Check sheet for the modelled part. Datum: model origin and axes. Units: mm. Face numbers are marked on the shaded views. A direction names the side the tool comes from. Coordinates: 2 decimals unless noted, no trailing zeros. Write each loop counter-clockwise with the first axis right and the second up, starting at its lowest first coordinate (ties: lowest second). Pieces come first, ordered by that corner, then holes. Notation, with made-up numbers: (52, 51) - (90, 51) arc R30 ccw to (90, 86) - close; hole circle Ø2 at (30, 54). An arc over 180 degrees is marked (long way). Answer as CSV lines item,"result". Start each with the question number.
from build123d import *

# Parameters (mm, degrees)
SKETCH2_W           = 38.1
SKETCH2_H           = 38.1
BOSS_EXTRUDE1_DEPTH = 5.08
SKETCH3_W           = 22.0218
SKETCH3_H           = 38.1
BOSS_EXTRUDE2_DEPTH = 5.08
SKETCH4_W           = 22.0218
SKETCH4_H           = 38.1
BOSS_EXTRUDE3_DEPTH = 5.08
SKETCH5_W           = 38.1
SKETCH5_H           = 38.1
BOSS_EXTRUDE4_DEPTH = 5.08
SKETCH6_R           = 4.826
CUT_EXTRUDE1_DEPTH  = 87.664926553
SKETCH7_R           = 4.826
CUT_EXTRUDE2_DEPTH  = 87.664926553
FILLET1_R           = 2.54
FILLET2_R           = 2.54
FILLET3_R           = 2.54
FILLET4_R           = 2.54
FILLET5_R           = 2.54


with BuildPart() as part:
    # Sketch2 → Boss-Extrude1 (new body)
    with BuildSketch(Plane.XY):
        with Locations((19.05, 19.05)):
            Rectangle(SKETCH2_W, SKETCH2_H)
    extrude(amount=-BOSS_EXTRUDE1_DEPTH)

    # Sketch3 → Boss-Extrude2 (add)
    with BuildSketch(Plane(origin=(38.1, 0, 0), x_dir=(0, 0, -1), z_dir=(1, 0, 0))):
        with Locations((11.0109, 19.05)):
            Rectangle(SKETCH3_W, SKETCH3_H)
    extrude(amount=-BOSS_EXTRUDE2_DEPTH)

    # Sketch4 → Boss-Extrude3 (add)
    with BuildSketch(Plane(origin=(0, 0, -22.0218), x_dir=(-1, 0, 0), z_dir=(0, 0, -1))):
        with Locations((-44.0309, 19.05)):
            Rectangle(SKETCH4_W, SKETCH4_H)
    extrude(amount=-BOSS_EXTRUDE3_DEPTH)

    # Sketch5 → Boss-Extrude4 (add)
    with BuildSketch(Plane(origin=(55.0418, 0, 0), x_dir=(0, 0, -1), z_dir=(1, 0, 0))):
        with Locations((35.9918, 19.05)):
            Rectangle(SKETCH5_W, SKETCH5_H)
    extrude(amount=-BOSS_EXTRUDE4_DEPTH)

    # Sketch6 → Cut-Extrude1 (cut, through all)
    with BuildSketch(Plane(origin=(55.0418, 0, 0), x_dir=(0, 0, -1), z_dir=(1, 0, 0))):
        with Locations((39.8018, 28.575)):
            Circle(SKETCH6_R)
        with Locations(Location((39.8018, 9.525, 0), (0, 0, 180))):
            Circle(SKETCH6_R)
    extrude(amount=-CUT_EXTRUDE1_DEPTH, mode=Mode.SUBTRACT)

    # Sketch7 → Cut-Extrude2 (cut, through all)
    with BuildSketch(Plane.XY):
        with Locations((15.24, 28.575)):
            Circle(SKETCH7_R)
        with Locations(Location((15.24, 9.525, 0), (0, 0, 180))):
            Circle(SKETCH7_R)
    extrude(amount=-CUT_EXTRUDE2_DEPTH, mode=Mode.SUBTRACT)

    # Fillet1
    fillet1_edges = [part.edges().sort_by_distance(p)[0] for p in [
        (49.9618, 19.05, -55.0418),
    ]]
    fillet(fillet1_edges, radius=FILLET1_R)

    # Fillet2
    fillet2_edges = [part.edges().sort_by_distance(p)[0] for p in [
        (49.9618, 19.05, -22.0218),
    ]]
    fillet(fillet2_edges, radius=FILLET2_R)

    # Fillet3
    fillet3_edges = [part.edges().sort_by_distance(p)[0] for p in [
        (33.02, 19.05, -22.0218),
    ]]
    fillet(fillet3_edges, radius=FILLET3_R)

    # Fillet4
    fillet4_edges = [part.edges().sort_by_distance(p)[0] for p in [
        (33.02, 19.05, -5.08),
    ]]
    fillet(fillet4_edges, radius=FILLET4_R)

    # Fillet5
    fillet5_edges = [part.edges().sort_by_distance(p)[0] for p in [
        (0, 19.05, -5.08),
    ]]
    fillet(fillet5_edges, radius=FILLET5_R)


solid = part.part
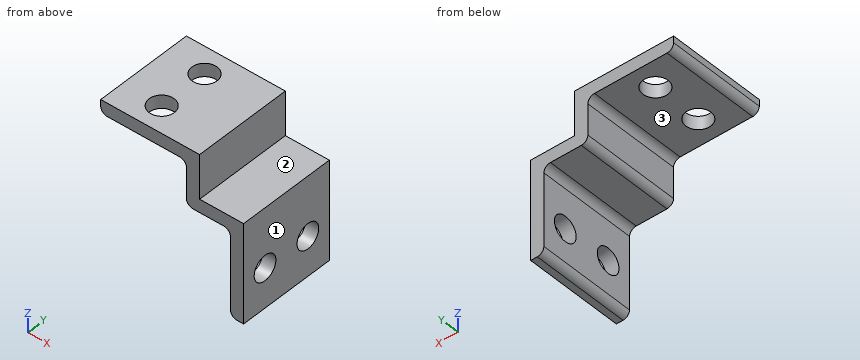
(1) Tool access check on the marked faces 1, 2 and 3. Record the directions out of +Z, -Z, +X, -X, +Y, -Y that give a thin tool (end or side, any length) a straight path to the whole face; none if there is none.
(2) Cross-section at B-B on y = 36. Record the boundary of the cut face in (x, z), plus the area to 3 significant figures.
(3) Cross-section at A-A on x = 15.24. Record the boundary of the cut face in (y, z), plus the area to 3 significant figures.
(4) Go/stop test with flat-tipped pins: P1, Ø12, axis at x = 44, z = -11, coming from the +Y side; P2, Ø12, axis at x = 32, y = 21.5, coming from the -Z side; P3, Ø7.5, axis at x = 15.24, y = 28.575, coming from the -Z side (3 decimals); P4, Ø3, axis at x = 43, y = 11, coming from the +Z side. Record where each tip stops, or that it passes through.
(5) Material ranges on probe 1 along Y at (x, z) = (15.24, -3); probe 2 along X at (y, z) = (13.5, -14.5), recorded low to high. Write a range as from..to.
(6) Cross-section at C-C on y = 25.5. Record the boundary of the cut face in (x, z), plus the area to 3 significant figures.
(7) Cross-section at D-D on x = 46. Record the boundary of the cut face in (y, z), plus the area to 3 significant figures.
Checked values:
1,face 1,"+Z, -Z, +X, +Y, -Y"
1,face 2,"+Z, +X, +Y, -Y"
1,face 3,"-Z, -X, +Y, -Y"
2,outline,"(0, -2.54) arc R2.54 ccw to (2.54, -5.08) - (30.48, -5.08) arc R2.54 cw to (33.02, -7.62) - (33.02, -19.48) arc R2.54 ccw to (35.56, -22.02) - (47.42, -22.02) arc R2.54 cw to (49.96, -24.56) - (49.96, -52.5) arc R2.54 ccw to (52.5, -55.04) - (55.04, -55.04) - (55.04, -16.94) - (38.1, -16.94) - (38.1, 0) - (0, 0) - close"
2,area,"532 mm^2"
3,outline,"(0, -5.08) - (4.7, -5.08) - (4.7, 0) - (0, 0) - close; (14.35, -5.08) - (23.75, -5.08) - (23.75, 0) - (14.35, 0) - close; (33.4, -5.08) - (38.1, -5.08) - (38.1, 0) - (33.4, 0) - close"
3,area,"95.5 mm^2"
4,P1,"y = 38.1"
4,P2,"z = -22.02"
4,P3,"through"
4,P4,"z = -16.94"
5,probe 1,"0..4.7, 14.35..23.75, 33.4..38.1"
5,probe 2,"33.02..38.1"
6,outline,"(0, -2.54) arc R2.54 ccw to (2.54, -5.08) - (11.52, -5.08) - (11.52, 0) - (0, 0) - close; (18.96, -5.08) - (30.48, -5.08) arc R2.54 cw to (33.02, -7.62) - (33.02, -19.48) arc R2.54 ccw to (35.56, -22.02) - (47.42, -22.02) arc R2.54 cw to (49.96, -24.56) - (49.96, -36.08) - (55.04, -36.08) - (55.04, -16.94) - (38.1, -16.94) - (38.1, 0) - (18.96, 0) - close; (49.96, -52.5) arc R2.54 ccw to (52.5, -55.04) - (55.04, -55.04) - (55.04, -43.52) - (49.96, -43.52) - close"
6,area,"456 mm^2"
7,outline,"(0, -22.02) - (38.1, -22.02) - (38.1, -16.94) - (0, -16.94) - close"
7,area,"194 mm^2"
